from build123d import *

# Parameters (mm, degrees)
BOSS_EXTRUDE1_DEPTH      = 35
BOSS_EXTRUDE2_DEPTH      = 35
FILLET1_R                = 0.5
SKETCH3_W                = 26
SKETCH3_H                = 25
CUT_EXTRUDE1_DEPTH       = 1.5
SKETCH4_W                = 16
SKETCH4_H                = 25
CUT_EXTRUDE2_DEPTH       = 5
FILLET3_R                = 1
SKETCH5_W                = 26
SKETCH5_H                = 25
CUT_EXTRUDE3_DEPTH       = 1.5
SKETCH6_W                = 16
SKETCH6_H                = 25
CUT_EXTRUDE4_DEPTH       = 5
FILLET4_R                = 1
SKETCH8_W                = 20
SKETCH8_H                = 3
CUT_EXTRUDE5_DEPTH       = 4
SKETCH9_W                = 20
SKETCH9_H                = 3
CUT_EXTRUDE6_DEPTH       = 4
SKETCH10_W               = 20
SKETCH10_H               = 3
CUT_EXTRUDE7_DEPTH       = 4
SKETCH11_R               = 1.1
CUT_EXTRUDE8_DEPTH       = 10
SKETCH12_R               = 1.1
CUT_EXTRUDE9_DEPTH       = 5
BOSS_EXTRUDE3_DEPTH      = 3.5
BOSS_EXTRUDE3_DEPTH_BACK = 1
SKETCH14_W               = 35
SKETCH14_H               = 3.801557548
SKETCH15_W               = 1.5
SKETCH15_H               = 31
CUT_EXTRUDE10_DEPTH      = 5
SKETCH18_W               = 35
SKETCH18_H               = 30
SKETCH18_R               = 1.1
SKETCH18_W_2             = 16
SKETCH18_H_2             = 20
BOSS_EXTRUDE4_DEPTH      = 6.5
SKETCH19_W               = 35
SKETCH19_H               = 30.5
SKETCH19_R               = 1.1
SKETCH19_W_2             = 16
SKETCH19_H_2             = 17.5
BOSS_EXTRUDE5_DEPTH      = 6.5
CUT_EXTRUDE12_DEPTH      = 2.5
CUT_EXTRUDE12_DEPTH_BACK = 10
SKETCH20_W               = 93.401628658
SKETCH20_H               = 53.255346894
SKETCH21_W               = 5
SKETCH21_H               = 4
CUT_EXTRUDE13_DEPTH      = 5.125
FILLET9_R                = 2
FILLET10_R               = 2
BOSS_EXTRUDE8_DEPTH      = 35


with BuildPart() as part:
    # Sketch1 → Boss-Extrude1 (new body)
    with BuildSketch(Plane.XY):
        Polygon((6.55, 4.55), (-6.55, 4.55), (-6.55, -4.55), (-2.05, -4.55), (-2.05, -2.05), (-4.05, -2.05), (-4.05, 2.05), (4.05, 2.05), (4.05, -2.05), (2.05, -2.05), (2.05, -4.55), (6.55, -4.55), align=None)
    extrude(amount=BOSS_EXTRUDE1_DEPTH)

    # Sketch2 → Boss-Extrude2 (add, through all)
    with BuildSketch(Plane.XY.offset(35)):
        Polygon((2.5, 4.55), (2.5, 25.721572875), (33.234018716, 56.455591591), (30.405591591, 59.284018716), (0.532284417, 29.410711541), (-18.64755944, 67.053274588), (-22.211585537, 65.237312589), (-2.5, 26.551147735), (-2.5, 4.55), align=None)
    extrude(amount=-BOSS_EXTRUDE2_DEPTH)

    # Fillet1
    fillet1_edges = [part.edges().sort_by_distance(p)[0] for p in [
        (0.532284417, 29.410711541, 17.5),
    ]]
    fillet(fillet1_edges, radius=FILLET1_R)

    # Sketch3 → Cut-Extrude1 (cut)
    with BuildSketch(Plane(origin=(-14.439213562, 14.439213562, 0), x_dir=(0, 0, 1), z_dir=(-0.7071067811865464, 0.7071067811865488, 0))):
        with Locations((17.5, 47.92013165)):
            Rectangle(SKETCH3_W, SKETCH3_H)
    extrude(amount=-CUT_EXTRUDE1_DEPTH, mode=Mode.SUBTRACT)

    # Sketch4 → Cut-Extrude2 (cut)
    with BuildSketch(Plane(origin=(-13.378553391, 13.378553391, 0), x_dir=(0, 0, 1), z_dir=(-0.7071067811865461, 0.707106781186549, 0))):
        with Locations((17.5, 47.92013165)):
            Rectangle(SKETCH4_W, SKETCH4_H)
    extrude(amount=-CUT_EXTRUDE2_DEPTH, mode=Mode.SUBTRACT)

    # Fillet3
    fillet3_edges = [part.edges().sort_by_distance(p)[0] for p in [
        (30.228814896, 55.218154724, 9.5),
        (30.228814896, 55.218154724, 25.5),
        (12.551145366, 37.540485194, 25.5),
        (12.551145366, 37.540485194, 9.5),
    ]]
    fillet(fillet3_edges, radius=FILLET3_R)

    # Sketch5 → Cut-Extrude3 (cut)
    with BuildSketch(Plane(origin=(12.3194594, 6.277078088, 0), x_dir=(0, 0, -1), z_dir=(0.8910065241883675, 0.45399049973954786, 0))):
        with Locations((-17.5, 52.710719955)):
            Rectangle(SKETCH5_W, SKETCH5_H)
    extrude(amount=-CUT_EXTRUDE3_DEPTH, mode=Mode.SUBTRACT)

    # Sketch6 → Cut-Extrude4 (cut)
    with BuildSketch(Plane(origin=(10.982949614, 5.596092339, 0), x_dir=(0, 0, -1), z_dir=(0.8910065241883673, 0.4539904997395479, 0))):
        with Locations((-17.5, 52.710719955)):
            Rectangle(SKETCH6_W, SKETCH6_H)
    extrude(amount=-CUT_EXTRUDE4_DEPTH, mode=Mode.SUBTRACT)

    # Fillet4
    fillet4_edges = [part.edges().sort_by_distance(p)[0] for p in [
        (-19.735855882, 63.131781141, 25.5),
        (-19.735855882, 63.131781141, 9.5),
        (-8.386093389, 40.856618036, 9.5),
        (-8.386093389, 40.856618036, 25.5),
    ]]
    fillet(fillet4_edges, radius=FILLET4_R)

    # Sketch8 → Cut-Extrude5 (cut)
    with BuildSketch(Plane(origin=(-11.610786438, 11.610786438, 0), x_dir=(0, 0, -1), z_dir=(0.7071067811865465, -0.7071067811865487, 0))):
        with Locations((-17.5, 29.42013165)):
            Rectangle(SKETCH8_W, SKETCH8_H)
    extrude(amount=-CUT_EXTRUDE5_DEPTH, mode=Mode.SUBTRACT)

    # Sketch9 → Cut-Extrude6 (cut)
    with BuildSketch(Plane(origin=(8.755433303, 4.461116089, 0), x_dir=(0, 0, 1), z_dir=(-0.8910065241883675, -0.45399049973954797, 0))):
        with Locations((17.5, 34.210719955)):
            Rectangle(SKETCH9_W, SKETCH9_H)
    extrude(amount=-CUT_EXTRUDE6_DEPTH, mode=Mode.SUBTRACT)

    # Sketch10 → Cut-Extrude7 (cut)
    with BuildSketch(Plane.ZY.offset(2.5)):
        with Locations((17.5, 19.55)):
            Rectangle(SKETCH10_W, SKETCH10_H)
    extrude(amount=-CUT_EXTRUDE7_DEPTH, mode=Mode.SUBTRACT)

    # Sketch11 → Cut-Extrude8 (cut)
    with BuildSketch(Plane(origin=(-13.378553391, 13.378553391, 0), x_dir=(0, 0, 1), z_dir=(-0.7071067811865461, 0.707106781186549, 0))):
        with Locations(Location((28, 57.92013165, 0), (0, 0, 270))):
            Circle(SKETCH11_R)
        with Locations(Location((7, 57.92013165, 0), (0, 0, 270))):
            Circle(SKETCH11_R)
        with Locations(Location((28, 45.42013165, 0), (0, 0, 270))):
            Circle(SKETCH11_R)
        with Locations(Location((7, 45.42013165, 0), (0, 0, 270))):
            Circle(SKETCH11_R)
    extrude(amount=-CUT_EXTRUDE8_DEPTH, mode=Mode.SUBTRACT)

    # Sketch12 → Cut-Extrude9 (cut)
    with BuildSketch(Plane(origin=(10.982949614, 5.596092339, 0), x_dir=(0, 0, -1), z_dir=(0.8910065241883673, 0.4539904997395479, 0))):
        with Locations(Location((-7, 62.710719955, 0), (0, 0, 90))):
            Circle(SKETCH12_R)
        with Locations(Location((-28, 62.710719955, 0), (0, 0, 90))):
            Circle(SKETCH12_R)
        with Locations(Location((-7, 50.210719955, 0), (0, 0, 90))):
            Circle(SKETCH12_R)
        with Locations(Location((-28, 50.210719955, 0), (0, 0, 90))):
            Circle(SKETCH12_R)
    extrude(amount=-CUT_EXTRUDE9_DEPTH, mode=Mode.SUBTRACT)

    # Sketch14 → Boss-Extrude3 (add, two sides: drawn at the far end of the back side and taken through both)
    with BuildSketch(Plane(origin=(6.55, 0, 0), x_dir=(0, 0, -1), z_dir=(1, 0, 0)).offset(-BOSS_EXTRUDE3_DEPTH_BACK)):
        with Locations((-17.5, -0.05)):
            Rectangle(SKETCH14_W, SKETCH14_H)
    extrude(amount=BOSS_EXTRUDE3_DEPTH + BOSS_EXTRUDE3_DEPTH_BACK)

    # Sketch15 → Cut-Extrude10 (cut)
    with BuildSketch(Plane(origin=(0, 1.850778774, 0), x_dir=(1, 0, 0), z_dir=(0, 1, 0))):
        with Locations((7.3, -17.5)):
            Rectangle(SKETCH15_W, SKETCH15_H)
    extrude(amount=-CUT_EXTRUDE10_DEPTH, mode=Mode.SUBTRACT)

    # Sketch18 → Boss-Extrude4 (add)
    with BuildSketch(Plane(origin=(-11.610786438, 11.610786438, 0), x_dir=(0, 0, -1), z_dir=(0.7071067811865465, -0.7071067811865487, 0))):
        with Locations((-17.5, 48.42013165)):
            Rectangle(SKETCH18_W, SKETCH18_H)
        with Locations(Location((-7, 57.92013165, 0), (0, 0, 270))):
            Circle(SKETCH18_R, mode=Mode.SUBTRACT)
        with Locations(Location((-7, 45.42013165, 0), (0, 0, 270))):
            Circle(SKETCH18_R, mode=Mode.SUBTRACT)
        with Locations(Location((-28, 45.42013165, 0), (0, 0, 270))):
            Circle(SKETCH18_R, mode=Mode.SUBTRACT)
        with Locations(Location((-28, 57.92013165, 0), (0, 0, 270))):
            Circle(SKETCH18_R, mode=Mode.SUBTRACT)
        with Locations((-17.5, 48.92013165)):
            Rectangle(SKETCH18_W_2, SKETCH18_H_2, mode=Mode.SUBTRACT)
    extrude(amount=BOSS_EXTRUDE4_DEPTH)

    # Sketch19 → Boss-Extrude5 (add)
    with BuildSketch(Plane(origin=(8.755433303, 4.461116089, 0), x_dir=(0, 0, 1), z_dir=(-0.8910065241883673, -0.45399049973954797, 0))):
        with Locations((17.5, 52.960719955)):
            Rectangle(SKETCH19_W, SKETCH19_H)
        with Locations(Location((28, 50.210719955, 0), (0, 0, 90))):
            Circle(SKETCH19_R, mode=Mode.SUBTRACT)
        with Locations(Location((7, 50.210719955, 0), (0, 0, 90))):
            Circle(SKETCH19_R, mode=Mode.SUBTRACT)
        with Locations(Location((7, 62.710719955, 0), (0, 0, 90))):
            Circle(SKETCH19_R, mode=Mode.SUBTRACT)
        with Locations(Location((28, 62.710719955, 0), (0, 0, 90))):
            Circle(SKETCH19_R, mode=Mode.SUBTRACT)
        with Locations((17.5, 51.960719955)):
            Rectangle(SKETCH19_W_2, SKETCH19_H_2, mode=Mode.SUBTRACT)
    extrude(amount=BOSS_EXTRUDE5_DEPTH)

    # Sketch20 → Cut-Extrude12 (cut, two sides: drawn at the far end of the back side and taken through both)
    with BuildSketch(Plane(origin=(0, 4.55, 0), x_dir=(1, 0, 0), z_dir=(0, 1, 0)).offset(-CUT_EXTRUDE12_DEPTH_BACK)):
        with Locations((0, -16.396538254)):
            Rectangle(SKETCH20_W, SKETCH20_H)
    extrude(amount=CUT_EXTRUDE12_DEPTH + CUT_EXTRUDE12_DEPTH_BACK, mode=Mode.SUBTRACT)

    # Sketch21 → Cut-Extrude13 (cut)
    with BuildSketch(Plane.XY.offset(35)):
        with Locations((0, 9.05)):
            Rectangle(SKETCH21_W, SKETCH21_H)
    cut_extrude13 = extrude(amount=-CUT_EXTRUDE13_DEPTH, mode=Mode.SUBTRACT)

    # Mirror1: Cut-Extrude13 across plane
    add(cut_extrude13.mirror(Plane(origin=(0, 0, 17.5), x_dir=(1, 0, 0), z_dir=(0, 0, -1))), mode=Mode.SUBTRACT)

    # Fillet9
    fillet9_edges = [part.edges().sort_by_distance(p)[0] for p in [
        (-21.702427992, 57.079294533, 9.5),
        (-13.757594247, 41.48668036, 9.5),
        (-13.757594247, 41.48668036, 25.5),
        (-21.702427992, 57.079294533, 25.5),
    ]]
    fillet(fillet9_edges, radius=FILLET9_R)

    # Fillet10
    fillet10_edges = [part.edges().sort_by_distance(p)[0] for p in [
        (32.350135239, 50.975514037, 25.5),
        (18.207999616, 36.833378413, 25.5),
        (18.207999616, 36.833378413, 9.5),
        (32.350135239, 50.975514037, 9.5),
    ]]
    fillet(fillet10_edges, radius=FILLET10_R)

    # Sketch25 → Boss-Extrude8 (add, through all)
    with BuildSketch(Plane.XY.offset(35)):
        Polygon((1.085786438, 24.307359313), (14.343145751, 11.05), (20, 11.05), (3.093757121, 27.956242879), align=None)
        Polygon((-2.594584578, 29.284990281), (-20.829574859, 11.05), (-15.17272061, 11.05), (-1.085786438, 25.136934172), align=None)
    extrude(amount=-BOSS_EXTRUDE8_DEPTH)


solid = part.part
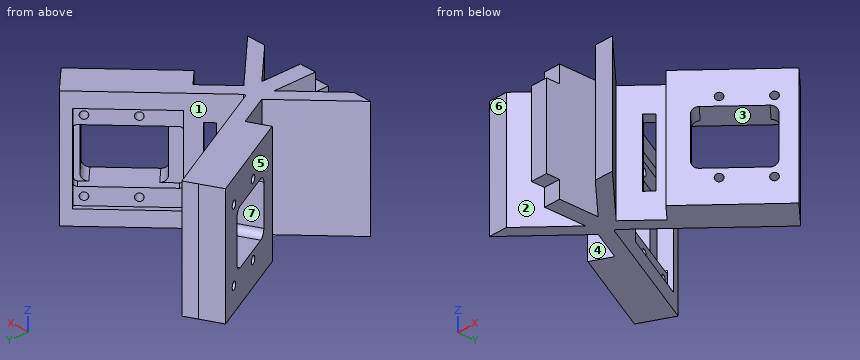
Build history of the part. All positions in model axes, mm. Face numbers are marked on the shaded views. A direction names the side the tool comes from. Give positions to 0.01 mm unless a question says otherwise; leave off trailing zeros. Loops run counter-clockwise (first coordinate to the right, second up) from the corner with the lowest first, then second, coordinate; pieces in that order, holes last. Notation, with made-up numbers: (1.25, 0) -> (28.25, 0) arc R4 ccw to (28.25, 7) -> close; hole circle Ø4 at (73.25, 73.5). An arc over 180 degrees is marked (long way). Answer in a Markdown table with one row per item.
Item 1: Mould opens along Y. For the marked faces 5, 6 and 7 say: pulls with the +Y half, pulls with the -Y half, needs draft (parallel to the pull), parting line crosses it, or undercut.
Findings below:
| item | result |
|---|---|
| face 5 | undercut |
| face 6 | pulls with the -Y half |
| face 7 | pulls with the +Y half |
Item 2: Flat gauge pins, fed straight in: P1, Ø1, axis at y = 51, z = 28.5, coming from the -X side; P2, Ø3, axis at x = 29, z = 5, coming from the +Y side; P3, Ø1, axis at y = 26, z = 18.5, coming from the -X side. Where does each tip first touch, or does it go through?
Findings below:
| item | result |
|---|---|
| P1 | stops at x = -22.51 |
| P2 | stops at y = 59.28 |
| P3 | stops at x = -6.38 |
Item 3: Slice it at A-A on y = 14. Write the cut outline in (x, z), plus the area to 3 significant figures.
Findings below:
| item | result |
|---|---|
| outline | (-17.88, 0) -> (-12.22, 0) -> (-12.22, 35) -> (-17.88, 35) -> close; (-2.5, 0) -> (2.5, 0) -> (2.5, 35) -> (-2.5, 35) -> close; (11.39, 0) -> (17.05, 0) -> (17.05, 35) -> (11.39, 35) -> close |
| area | 571 mm² |
Item 4: Tool access for the marked faces 1, 2, 3 and 4: list every direction of +Z, -Z, +X, -X, +Y, -Y with a clear straight run to the whole face (end or side of a thin tool).
Findings below:
| item | result |
|---|---|
| face 1 | +Z, -Z, +Y |
| face 2 | +Z, -Z, -Y |
| face 3 | none |
| face 4 | +Z, -Z |
Item 5: Slice it at D-D on y = 26. Write the cut outline in (x, z), plus the area to 3 significant figures.
Findings below:
| item | result |
|---|---|
| outline | (-5.88, 0) -> (5.05, 0) -> (5.05, 35) -> (-5.88, 35) -> close |
| area | 383 mm² |
Item 6: Slice it at B-B on x = -1.5. Write the cut outline in (y, z) (3 decimals).
Findings below:
| item | result |
|---|---|
| outline | (7.05, 5.125) -> (11.05, 5.125) -> (11.05, 0) -> (33.399, 0) -> (33.399, 35) -> (11.05, 35) -> (11.05, 29.875) -> (7.05, 29.875) -> close; hole (18.05, 7.5) -> (21.05, 7.5) -> (21.05, 27.5) -> (18.05, 27.5) -> close |
Item 7: Probe line 1 along Z through (x, y) = (28.5, 53.5); line 2 along Y through (x, z) = (-19, 22); line 3 along Z through (x, y) = (25.5, 50.5). List the from-to ranges inside material, lowest first. Write a range as [from, to].
Findings below:
| item | result |
|---|---|
| line 1 | z = [0, 5.9], [8.1, 9.5], [25.5, 26.9], [29.1, 35] |
| line 2 | y = [11.05, 12.88], [58.46, 58.93], [63.51, 66.87] |
| line 3 | z = [0, 9.5], [25.5, 35] |
Item 8: Slice it at C-C on z = 15. Give the number of separate pieces and of enclosed holes in the cut face, plus the area to 3 significant figures.
Findings below:
| item | result |
|---|---|
| separate pieces | 5 |
| enclosed holes | 0 |
| area | 528 mm² |
